Can you work these out from the model? Positions are in its coordinate system, mm. Face numbers are marked on the shaded views. A direction names the side the tool comes from. Give positions to 0.01 mm unless a question says otherwise; leave off trailing zeros. Write each loop counter-clockwise with the first axis right and the second up, starting at its lowest first coordinate (ties: lowest second). Pieces come first, ordered by that corner, then holes. Notation, with made-up numbers: (7, 3.25) -> (60, 3.25) arc R23 cw to (60, 27.25) -> close; hole circle Ø3 at (1, 70). An arc over 180 degrees is marked (long way). Answer as CSV lines item,"result". Start each with the question number.
1. If we section it at D-D on x = 2: Write out the boundary of the cut face in (y, z), plus the area to 3 significant figures.
2. If we section it at A-A on z = 0: Write out the boundary of the cut face in (x, y).
3. If we section it at C-C on x = -11.5: Write out the boundary of the cut face in (y, z), plus the area to 3 significant figures.
4. I need wall thicknesses on line 1 (Y direction, x = 8, z = 10); line 2 (Y direction, x = -2, z = 0); line 3 (Z direction, x = -5, y = 0). Which ranges of each line are inside material? Lowest first, please. Write a range as [from, to].
5. On a 3-axis mill with a long thin cutter (end or side, diameter ignored), from which of +Z, -Z, +X, -X, +Y, -Y can I reach the whole of each face in a straight line? I mean the marked faces 1, 2 and 3. Say none if no direction works.
6. I'm going to push flat-ended pins straight in: P1, Ø8, axis at x = -2.5, z = -8, coming from the +Y side; P2, Ø1, axis at y = 79, z = 7, coming from the -X side; P3, Ø8, axis at y = 48.5, z = -56, coming from the -X side. Where does each tip first touch, or does it pass through?
7. If we section it at B-B on y = 0: Write out the boundary of the cut face in (x, z), plus the area to 4 significant figures.
8. If we mould it in two halves opening along Z, with no side actions, what happens to the marked faces 4, 5, 6 and 7? For each: pulls with the +Z half, pulls with the -Z half, needs draft (parallel to the pull), parting line crosses it, or undercut.
```python
from build123d import *

# Parameters (mm, degrees)
F3_DEPTH = 40.001


with BuildPart() as f1:
    # F0 (on Front) → F1 (revolve)
    with BuildSketch(Plane.XZ):
        Polygon((-20, 25), (0, 25), (20, 25), (20, 35), (7.5, 40), (7.5, 70), (19, 80), (19, 100), (0, 100), (-19, 100), (-19, 80), (-7.5, 70), (-7.5, 40), (-20, 35), align=None)
    revolve(axis=Axis((21.959458, 0, 0), (1, 0, 0)))

    # F2 (on face) → F3 (cut, through all)
    with BuildSketch(Plane.YZ.offset(20)):
        with BuildLine():
            Line((7, 24), (7, 30))
            Line((7, 30), (-7, 30))
            Line((-7, 30), (-7, 24))
            ThreePointArc((-7, 24), (0, 25), (7, 24))
        make_face()
    extrude(amount=-F3_DEPTH, mode=Mode.SUBTRACT)


solid = f1.part
```
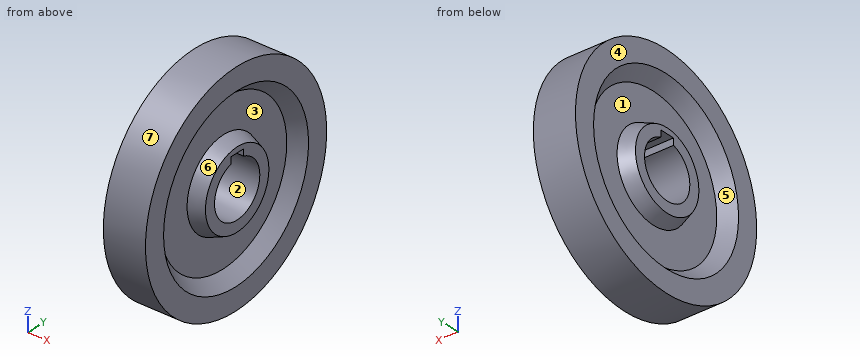
Computed values:
1,outline,"circle Ø200 at (0, 0); hole (-7, 24) arc R25 ccw (long way) to (7, 24) -> (7, 30) -> (-7, 30) -> close"
1,area,"29,400 mm2"
2,outline,"(-20, -35) -> (-7.5, -40) -> (-7.5, -70) -> (-19, -80) -> (-19, -100) -> (19, -100) -> (19, -80) -> (7.5, -70) -> (7.5, -40) -> (20, -35) -> (20, -25) -> (-20, -25) -> close; (-20, 25) -> (20, 25) -> (20, 35) -> (7.5, 40) -> (7.5, 70) -> (19, 80) -> (19, 100) -> (-19, 100) -> (-19, 80) -> (-7.5, 70) -> (-7.5, 40) -> (-20, 35) -> close"
3,outline,"circle Ø200 at (0, 0); circle Ø76.8 at (0, 0); hole circle Ø146.96 at (0, 0); hole (-7, 24) arc R25 ccw (long way) to (7, 24) -> (7, 30) -> (-7, 30) -> close"
3,area,"17,000 mm2"
4,line 1,"y = [-99.5, -69.72], [-38.52, -22.91], [22.91, 38.52], [69.72, 99.5]"
4,line 2,"y = [-100, -25], [25, 100]"
4,line 3,"z = [-100, -25], [30, 100]"
5,face 1,"-X"
5,face 2,"+X, -X"
5,face 3,"+X"
6,P1,"stops at y = 99.92"
6,P2,"stops at x = -18.78"
6,P3,"stops at x = -16.8"
7,outline,"(-20, -35) -> (-7.5, -40) -> (-7.5, -70) -> (-19, -80) -> (-19, -100) -> (19, -100) -> (19, -80) -> (7.5, -70) -> (7.5, -40) -> (20, -35) -> (20, -25) -> (-20, -25) -> close; (-20, 30) -> (20, 30) -> (20, 35) -> (7.5, 40) -> (7.5, 70) -> (19, 80) -> (19, 100) -> (-19, 100) -> (-19, 80) -> (-7.5, 70) -> (-7.5, 40) -> (-20, 35) -> close"
7,area,"3,825 mm2"
8,face 4,"needs draft"
8,face 5,"undercut"
8,face 6,"undercut"
8,face 7,"parting line crosses it"
